Work out the finished part from the listing and answer in its coordinate system (mm). A direction names the side the tool comes from. Coordinates: 2 decimals unless noted, no trailing zeros. Order: outer loops, then holes, each group sorted by start corner. A loop starts at its lowest first (then second) coordinate and runs counter-clockwise, first axis right, second up. Notation, with made-up numbers: M 0.25,0.5 L 27.25,0.5 A17 cw 27.25,15.5 Z; hole C -26,79.5 d2. An arc over 180 degrees is marked long. Answer in a Markdown table with one row per item. Add a question column.
Item 1: The part is cut by section C-C (x = -27). Write down the section's boundary in (y, z), then the cut area to 3 significant figures.
Item 2: The mould has two halves that part along X. Classify faces 1 (the face through (-1.08, 0.07, -4.88)), 2 (the face through (6, 5, 0)), 3 (the face through (-16.49, 19.72, -30.87)), 4 (the face through (24, 0, 15)): released by +X, released by -X, zero draft, split by the parting line, or undercut.
Item 3: Flat-ended cylindrical pins translate along their axes: pin 1 Ø4 at (y, z) = (1, 8) entering from -X; pin 2 Ø1.5 at (y, z) = (14.5, 4) entering from -X; pin 3 Ø4 at (x, z) = (17.5, -23) entering from -Y; pin 4 Ø3 at (x, z) = (21, 20.5) entering from +Y. Find the tip coordinate at first contact, or state that the pin passes through.
Item 4: The part is cut by section B-B (z = -10). Write down the section's boundary in (x, y), then the cut area to 3 significant figures.
Item 5: The part is cut by section A-A (y = 2). State how many separate pieces and enclosed holes the cut face has, then the cut area to 3 significant figures.
Item 6: Consider line 1 (Z direction, x = 0, y = 2.5); line 2 (Y direction, x = 18, z = 27); line 3 (Y direction, x = 19.5, z = -12.5). Determine where each line is inside the solid, lowest interval first. Write a range as from..to.
Item 7: Which of the six approach directions +Z, -Z, +X, -X, +Y, -Y give full straight-line access (tool end or side, diameter ignored) to faces 5 (the face through (34.98, 19.72, 1.15)), 6 (the face through (25.865, 2.465, -10.724)), 7 (the face through (-1.08, 39.93, 4.88))?
Item 8: The part is cut by section D-D (z = 30.5). Write down the section's boundary in (x, y), then the cut area to 3 significant figures.
from build123d import *

# Parameters (mm, degrees)
BOSS_EXTRUDE1_DEPTH = 40
SKETCH2_R           = 28
CUT_EXTRUDE1_DEPTH  = 5
SKETCH3_R           = 28
CUT_EXTRUDE2_DEPTH  = 5
SKETCH4_R           = 5
BOSS_EXTRUDE2_DEPTH = 10
SKETCH5_R           = 5
BOSS_EXTRUDE3_DEPTH = 10
SKETCH6_R           = 3
CUT_EXTRUDE3_DEPTH  = 51


with BuildPart() as part:
    # Sketch1 → Boss-Extrude1 (new body)
    with BuildSketch(Plane(origin=(0, 0, 0), x_dir=(1, 0, 0), z_dir=(0, 1, 0))):
        with BuildLine():
            Line((-9.316786783, 33.737182515), (-9.183689829, 33.255222765))
            ThreePointArc((-9.183689829, 33.255222765), (-4.764444491, 34.169431788), (-0.263678186, 34.498992359))
            Line((-0.263678186, 34.498992359), (-0.267499609, 34.998977756))
            ThreePointArc((-0.267499609, 34.998977756), (7.314006433, 34.227259749), (14.548770163, 31.832896298))
            Line((14.548770163, 31.832896298), (14.340930589, 31.378140637))
            ThreePointArc((14.340930589, 31.378140637), (18.313911156, 29.237829231), (21.973535626, 26.597250461))
            Line((21.973535626, 26.597250461), (22.291992664, 26.982717859))
            ThreePointArc((22.291992664, 26.982717859), (27.603712465, 21.518249421), (31.606795859, 15.033644121))
            Line((31.606795859, 15.033644121), (31.155270204, 14.818877776))
            ThreePointArc((31.155270204, 14.818877776), (32.822984237, 10.625521435), (33.92908791, 6.250359477))
            Line((33.92908791, 6.250359477), (34.420813822, 6.340944397))
            ThreePointArc((34.420813822, 6.340944397), (34.977334653, -1.259388959), (33.875650502, -8.800017221))
            Line((33.875650502, -8.800017221), (33.391712637, -8.67430269))
            ThreePointArc((33.391712637, -8.67430269), (31.973818206, -12.95858593), (30.008842881, -17.021144172))
            Line((30.008842881, -17.021144172), (30.443753648, -17.267827421))
            ThreePointArc((30.443753648, -17.267827421), (25.984673227, -23.447745249), (20.293711789, -28.516052704))
            Line((20.293711789, -28.516052704), (20.00380162, -28.108680523))
            ThreePointArc((20.00380162, -28.108680523), (16.163747288, -30.47922692), (12.047126757, -32.328265294))
            Line((12.047126757, -32.328265294), (12.221722797, -32.796790878))
            ThreePointArc((12.221722797, -32.796790878), (4.833494411, -34.664640944), (-2.783880209, -34.889110206))
            Line((-2.783880209, -34.889110206), (-2.744110492, -34.390694346))
            ThreePointArc((-2.744110492, -34.390694346), (-7.209520627, -33.738298895), (-11.551573865, -32.508631796))
            Line((-11.551573865, -32.508631796), (-11.718987979, -32.979771387))
            ThreePointArc((-11.718987979, -32.979771387), (-18.579330159, -29.661565887), (-24.558863718, -24.937165293))
            Line((-24.558863718, -24.937165293), (-24.208022808, -24.580920075))
            ThreePointArc((-24.208022808, -24.580920075), (-27.209373716, -21.210845858), (-29.745164695, -17.477848187))
            Line((-29.745164695, -17.477848187), (-30.176254039, -17.731150335))
            ThreePointArc((-30.176254039, -17.731150335), (-33.298679661, -10.7795145), (-34.842481952, -3.316843594))
            Line((-34.842481952, -3.316843594), (-34.34473221, -3.269460114))
            ThreePointArc((-34.34473221, -3.269460114), (-34.477658444, 1.241397688), (-34.020662383, 5.731014832))
            Line((-34.020662383, 5.731014832), (-34.513715461, 5.814073018))
            ThreePointArc((-34.513715461, 5.814073018), (-32.437206876, 13.146391523), (-28.822915649, 19.855466085))
            Line((-28.822915649, 19.855466085), (-28.411159712, 19.57181657))
            ThreePointArc((-28.411159712, 19.57181657), (-25.61346361, 23.11277746), (-22.377514045, 26.258272319))
            Line((-22.377514045, 26.258272319), (-22.701825842, 26.63882699))
            ThreePointArc((-22.701825842, 26.63882699), (-16.398004495, 30.920954846), (-9.316786783, 33.737182515))
        make_face()
    extrude(amount=BOSS_EXTRUDE1_DEPTH)

    # Sketch2 → Cut-Extrude1 (cut)
    with BuildSketch(Plane(origin=(0, 40, 0), x_dir=(1, 0, 0), z_dir=(0, 1, 0))):
        Circle(SKETCH2_R)
    extrude(amount=-CUT_EXTRUDE1_DEPTH, mode=Mode.SUBTRACT)

    # Sketch3 → Cut-Extrude2 (cut)
    with BuildSketch(Plane.XZ):
        Circle(SKETCH3_R)
    extrude(amount=-CUT_EXTRUDE2_DEPTH, mode=Mode.SUBTRACT)

    # Sketch4 → Boss-Extrude2 (add)
    with BuildSketch(Plane(origin=(0, 35, 0), x_dir=(1, 0, 0), z_dir=(0, 1, 0))):
        Circle(SKETCH4_R)
    extrude(amount=BOSS_EXTRUDE2_DEPTH)

    # Sketch5 → Boss-Extrude3 (add)
    with BuildSketch(Plane.XZ.offset(-5)):
        Circle(SKETCH5_R)
    extrude(amount=BOSS_EXTRUDE3_DEPTH)

    # Sketch6 → Cut-Extrude3 (cut, through all)
    with BuildSketch(Plane.XZ.offset(5)):
        Circle(SKETCH6_R)
    extrude(amount=-CUT_EXTRUDE3_DEPTH, mode=Mode.SUBTRACT)


solid = part.part
Reply:
| question | item | result |
|---|---|---|
| 1 | outline | M 0,-21.48 L 40,-21.48 L 40,-7.42 L 35,-7.42 L 35,7.42 L 40,7.42 L 40,21.48 L 0,21.48 L 0,7.42 L 5,7.42 L 5,-7.42 L 0,-7.42 Z |
| 1 | area | 1,570 mm2 |
| 2 | face 1 | undercut |
| 2 | face 2 | undercut |
| 2 | face 3 | released by -X |
| 2 | face 4 | zero draft |
| 3 | pin 1 | stops at x = -34.48 |
| 3 | pin 2 | stops at x = -34.84 |
| 3 | pin 3 | stops at y = 0 |
| 3 | pin 4 | stops at y = 40 |
| 4 | outline | M -33.54,0 L -26.15,0 L -26.15,5 L 26.15,5 L 26.15,0 L 33.02,0 L 33.02,40 L 26.15,40 L 26.15,35 L -26.15,35 L -26.15,40 L -33.54,40 Z |
| 4 | area | 2,140 mm2 |
| 5 | separate pieces | 2 |
| 5 | enclosed holes | 2 |
| 5 | area | 1,390 mm2 |
| 6 | line 1 | z = -35..-28, -5..-3, 3..5, 28..35 |
| 6 | line 2 | y = 0..40 |
| 6 | line 3 | y = 5..35 |
| 7 | face 5 | +X, +Y, -Y |
| 7 | face 6 | -Y |
| 7 | face 7 | +Y |
| 8 | outline | M -17.17,0 L 16.12,0 L 16.12,40 L -17.17,40 Z |
| 8 | area | 1,330 mm2 |
